```python
from build123d import *

# Parameters (mm, degrees)
SKETCH1_W           = 412.75
SKETCH1_H           = 584.2
BOSS_EXTRUDE1_DEPTH = 4.7625
SKETCH2_W           = 40.64
SKETCH2_H           = 139.7
CUT_EXTRUDE1_DEPTH  = 716.314534947
SKETCH3_R           = 2.667
CUT_EXTRUDE2_DEPTH  = 254


with BuildPart() as part:
    # Sketch1 → Boss-Extrude1 (new body)
    with BuildSketch(Plane(origin=(0, 0, 0), x_dir=(1, 0, 0), z_dir=(0, 1, 0))):
        with Locations((206.375, 292.1)):
            Rectangle(SKETCH1_W, SKETCH1_H)
    extrude(amount=BOSS_EXTRUDE1_DEPTH)

    # Sketch2 → Cut-Extrude1 (cut, through all)
    with BuildSketch(Plane(origin=(0, 4.7625, 0), x_dir=(1, 0, 0), z_dir=(0, 1, 0))):
        with Locations((20.32, 407.162)):
            Rectangle(SKETCH2_W, SKETCH2_H)
        with Locations((392.43, 407.162)):
            Rectangle(SKETCH2_W, SKETCH2_H)
    extrude(amount=-CUT_EXTRUDE1_DEPTH, mode=Mode.SUBTRACT)

    # Sketch3 → Cut-Extrude2 (cut)
    with BuildSketch(Plane(origin=(0, 4.7625, 0), x_dir=(1, 0, 0), z_dir=(0, 1, 0))):
        with Locations(Location((9.525, 13.462, 0), (0, 0, 270))):
            Circle(SKETCH3_R)
        with Locations(Location((34.925, 13.462, 0), (0, 0, 270))):
            Circle(SKETCH3_R)
        with Locations(Location((60.325, 13.462, 0), (0, 0, 270))):
            Circle(SKETCH3_R)
        with Locations(Location((85.725, 13.462, 0), (0, 0, 270))):
            Circle(SKETCH3_R)
        with Locations(Location((111.125, 13.462, 0), (0, 0, 270))):
            Circle(SKETCH3_R)
        with Locations(Location((136.525, 13.462, 0), (0, 0, 270))):
            Circle(SKETCH3_R)
        with Locations(Location((161.925, 13.462, 0), (0, 0, 270))):
            Circle(SKETCH3_R)
        with Locations(Location((187.325, 13.462, 0), (0, 0, 270))):
            Circle(SKETCH3_R)
        with Locations(Location((225.425, 13.462, 0), (0, 0, 270))):
            Circle(SKETCH3_R)
        with Locations(Location((250.825, 13.462, 0), (0, 0, 270))):
            Circle(SKETCH3_R)
        with Locations(Location((276.225, 13.462, 0), (0, 0, 270))):
            Circle(SKETCH3_R)
        with Locations(Location((301.625, 13.462, 0), (0, 0, 270))):
            Circle(SKETCH3_R)
        with Locations(Location((327.025, 13.462, 0), (0, 0, 270))):
            Circle(SKETCH3_R)
        with Locations(Location((352.425, 13.462, 0), (0, 0, 270))):
            Circle(SKETCH3_R)
        with Locations(Location((377.825, 13.462, 0), (0, 0, 270))):
            Circle(SKETCH3_R)
        with Locations(Location((403.225, 13.462, 0), (0, 0, 270))):
            Circle(SKETCH3_R)
        with Locations(Location((403.225, 38.862, 0), (0, 0, 270))):
            Circle(SKETCH3_R)
        with Locations(Location((403.225, 64.262, 0), (0, 0, 270))):
            Circle(SKETCH3_R)
        with Locations(Location((403.225, 89.662, 0), (0, 0, 270))):
            Circle(SKETCH3_R)
        with Locations(Location((403.225, 115.062, 0), (0, 0, 270))):
            Circle(SKETCH3_R)
        with Locations(Location((403.225, 140.462, 0), (0, 0, 270))):
            Circle(SKETCH3_R)
        with Locations(Location((403.225, 165.862, 0), (0, 0, 270))):
            Circle(SKETCH3_R)
        with Locations(Location((403.225, 191.262, 0), (0, 0, 270))):
            Circle(SKETCH3_R)
        with Locations(Location((403.225, 216.662, 0), (0, 0, 270))):
            Circle(SKETCH3_R)
        with Locations(Location((403.225, 242.062, 0), (0, 0, 270))):
            Circle(SKETCH3_R)
        with Locations(Location((403.225, 267.462, 0), (0, 0, 270))):
            Circle(SKETCH3_R)
        with Locations(Location((403.225, 292.862, 0), (0, 0, 270))):
            Circle(SKETCH3_R)
        with Locations(Location((403.225, 318.262, 0), (0, 0, 270))):
            Circle(SKETCH3_R)
        with Locations((403.225, 343.662)):
            Circle(SKETCH3_R)
        with Locations((403.225, 369.062)):
            Circle(SKETCH3_R)
        with Locations((403.225, 394.462)):
            Circle(SKETCH3_R)
        with Locations((403.225, 419.862)):
            Circle(SKETCH3_R)
        with Locations((403.225, 445.262)):
            Circle(SKETCH3_R)
        with Locations((403.225, 470.662)):
            Circle(SKETCH3_R)
        with Locations(Location((403.225, 496.062, 0), (0, 0, 270))):
            Circle(SKETCH3_R)
        with Locations(Location((403.225, 521.462, 0), (0, 0, 270))):
            Circle(SKETCH3_R)
        with Locations(Location((403.225, 546.862, 0), (0, 0, 270))):
            Circle(SKETCH3_R)
        with Locations(Location((403.225, 572.262, 0), (0, 0, 270))):
            Circle(SKETCH3_R)
        with Locations(Location((9.525, 38.862, 0), (0, 0, 270))):
            Circle(SKETCH3_R)
        with Locations(Location((9.525, 64.262, 0), (0, 0, 270))):
            Circle(SKETCH3_R)
        with Locations(Location((9.525, 89.662, 0), (0, 0, 270))):
            Circle(SKETCH3_R)
        with Locations(Location((9.525, 115.062, 0), (0, 0, 270))):
            Circle(SKETCH3_R)
        with Locations(Location((9.525, 140.462, 0), (0, 0, 270))):
            Circle(SKETCH3_R)
        with Locations(Location((9.525, 165.862, 0), (0, 0, 270))):
            Circle(SKETCH3_R)
        with Locations(Location((9.525, 191.262, 0), (0, 0, 270))):
            Circle(SKETCH3_R)
        with Locations(Location((9.525, 216.662, 0), (0, 0, 270))):
            Circle(SKETCH3_R)
        with Locations(Location((9.525, 242.062, 0), (0, 0, 270))):
            Circle(SKETCH3_R)
        with Locations(Location((9.525, 267.462, 0), (0, 0, 270))):
            Circle(SKETCH3_R)
        with Locations(Location((9.525, 292.862, 0), (0, 0, 270))):
            Circle(SKETCH3_R)
        with Locations(Location((9.525, 318.262, 0), (0, 0, 270))):
            Circle(SKETCH3_R)
        with Locations((9.525, 343.662)):
            Circle(SKETCH3_R)
        with Locations((9.525, 369.062)):
            Circle(SKETCH3_R)
        with Locations((9.525, 394.462)):
            Circle(SKETCH3_R)
        with Locations((9.525, 419.862)):
            Circle(SKETCH3_R)
        with Locations((9.525, 445.262)):
            Circle(SKETCH3_R)
        with Locations((9.525, 470.662)):
            Circle(SKETCH3_R)
        with Locations(Location((9.525, 496.062, 0), (0, 0, 270))):
            Circle(SKETCH3_R)
        with Locations(Location((9.525, 521.462, 0), (0, 0, 270))):
            Circle(SKETCH3_R)
        with Locations(Location((9.525, 546.862, 0), (0, 0, 270))):
            Circle(SKETCH3_R)
        with Locations(Location((9.525, 572.262, 0), (0, 0, 270))):
            Circle(SKETCH3_R)
    extrude(amount=-CUT_EXTRUDE2_DEPTH, mode=Mode.SUBTRACT)


solid = part.part
```
Geometry check sheet. Reference: the model listing, model coordinates, mm. Coordinates: 2 decimals unless noted, no trailing zeros. Order: outer loops, then holes, each group sorted by start corner. A loop starts at its lowest first (then second) coordinate and runs counter-clockwise, first axis right, second up.
Q1. Sectioned sample at A-A on z = -443.5. Record the cut outline in (x, y), and give its area (3 significant figures).
Reply:
outline: (40.64, 0) - (372.11, 0) - (372.11, 4.76) - (40.64, 4.76) - close
area: 1,580 mm2
Q2. Depth check by flat-ended pin: pin 1 Ø2.5 at (y, z) = (1.5, -374.5) entering from -X. Enter the tip coordinate at first touch or a pass-through.
Reply:
pin 1: stops at x = 40.64
Q3. Thickness scan on probe 1 along X at (y, z) = (3.8, -320.5); probe 2 along X at (y, z) = (4.1, -290.5); probe 3 along Z at (x, y) = (189.5, 3.55). Record the ranges inside material, lowest first.
Reply:
probe 1: x = 0 to 8.07, 10.98 to 401.77, 404.68 to 412.75
probe 2: x = 0 to 8.29, 10.76 to 401.99, 404.46 to 412.75
probe 3: z = -584.2 to -15.01, -11.92 to 0
Q4. Sectioned sample at B-B on y = 3.6. Give the number of separate pieces and of enclosed holes in the cut face, and give its area (3 significant figures).
Reply:
separate pieces: 1
enclosed holes: 48
area: 229,000 mm2
